from build123d import *

# Parameters (mm, degrees)
SKETCH1_R           = 7
SKETCH1_R_2         = 5
BOSS_EXTRUDE1_DEPTH = 12
CUT_EXTRUDE1_DEPTH  = 40.522145691
FILLET1_R           = 1
BOSS_EXTRUDE2_START = -12
BOSS_EXTRUDE2_DEPTH = 12
FILLET2_R           = 2
CUT_EXTRUDE2_DEPTH  = 59.481408086
SKETCH7_R           = 1.5
CUT_EXTRUDE3_DEPTH  = 65.024019647


with BuildPart() as part:
    # Sketch1 → Boss-Extrude1 (new body)
    with BuildSketch(Plane(origin=(0, 0, 0), x_dir=(0, 0, -1), z_dir=(1, 0, 0))):
        with Locations((-30, 0)):
            Circle(SKETCH1_R)
        with Locations((-30, 0)):
            Circle(SKETCH1_R_2, mode=Mode.SUBTRACT)
    extrude(amount=BOSS_EXTRUDE1_DEPTH)

    # Sketch3 → Cut-Extrude1 (cut, through all)
    with BuildSketch(Plane(origin=(12, 0, 0), x_dir=(0, 0, -1), z_dir=(1, 0, 0))):
        Polygon((-26.132418273, 3.168881756), (-27.092472621, -4.067712446), (-40.54775296, -2.282646151), (-39.587698612, 4.953948051), align=None)
    extrude(amount=-CUT_EXTRUDE1_DEPTH, mode=Mode.SUBTRACT)

    # Fillet1
    fillet1_edges = [part.edges().sort_by_distance(p)[0] for p in [
        (6, 4.067712446, 32.907527379),
        (6, 4.403840469, 35.441156966),
        (6, -3.168881756, 33.867581727),
        (6, -2.832753733, 36.401211314),
    ]]
    fillet(fillet1_edges, radius=FILLET1_R - 0.0001)  # a hair under: the kernel refuses the full size

    # Sketch4 → Boss-Extrude2 (add)
    with BuildSketch(Plane(origin=(12, 0, 0), x_dir=(0, 0, -1), z_dir=(1, 0, 0)).offset(BOSS_EXTRUDE2_START)):
        with BuildLine():
            Line((-23.06080008, -0.92060006), (-17, 40))
            Line((-17, 40), (0, 40))
            Line((0, 40), (0, 45))
            Line((0, 45), (-23, 45))
            Line((-23, 45), (-32.940967226, 6.352221011))
            ThreePointArc((-32.940967226, 6.352221011), (-25.850307511, 5.63737991), (-23.06080008, -0.92060006))
        make_face()
    extrude(amount=BOSS_EXTRUDE2_DEPTH)

    # Fillet2
    fillet2_edges = [part.edges().sort_by_distance(p)[0] for p in [
        (6, 40, 17),
    ]]
    fillet(fillet2_edges, radius=FILLET2_R)

    # Sketch6 → Cut-Extrude2 (cut, through all)
    with BuildSketch(Plane(origin=(12, 0, 0), x_dir=(0, 0, -1), z_dir=(1, 0, 0))):
        with BuildLine():
            Line((-24.037943225, 10.910448491), (-21.102528553, 30.729437441))
            ThreePointArc((-21.102528553, 30.729437441), (-22.170547869, 32.250479964), (-23.74540162, 31.263529469))
            Line((-23.74540162, 31.263529469), (-28.73638424, 11.859945407))
            ThreePointArc((-28.73638424, 11.859945407), (-26.887444194, 8.909635204), (-24.037943225, 10.910448491))
        make_face()
    extrude(amount=-CUT_EXTRUDE2_DEPTH, mode=Mode.SUBTRACT)

    # Mirror9: part across plane


with BuildPart() as part_1:
    add(part.part)
    add(part.part.mirror(Plane(origin=(-56.513793287, 40, 0), x_dir=(1, 0, 0), z_dir=(0, 0, -1))))

    # Sketch7 → Cut-Extrude3 (cut, through all)
    with BuildSketch(Plane(origin=(0, 45, 0), x_dir=(1, 0, 0), z_dir=(0, 1, 0))):
        with Locations(Location((6, -12.5, 0), (0, 0, 270))):
            Circle(SKETCH7_R)
        with Locations(Location((6, 12.5, 0), (0, 0, 270))):
            Circle(SKETCH7_R)
    extrude(amount=-CUT_EXTRUDE3_DEPTH, mode=Mode.SUBTRACT)


solid = part_1.part
Here's how the part is built. I have some questions about the finished solid (model axes, mm). A direction names the side the tool comes from. Coordinates: 2 decimals unless noted, no trailing zeros. Write each loop counter-clockwise with the first axis right and the second up, starting at its lowest first coordinate (ties: lowest second). Pieces come first, ordered by that corner, then holes.
1) If we section it at C-C (y = 0): List the corners of the cut face in (x, z) for me.
Filled in:
outline: (0, -25) - (12, -25) - (12, -22.92) - (0, -22.92) - close; (0, 22.92) - (12, 22.92) - (12, 25) - (0, 25) - close
2) If I drill on line 1 (Z direction, x = 11, y = 25); line 2 (X direction, y = 43.9, z = 12.5); line 3 (Z direction, x = 9, y = 10.5), over which ranges is the centre line in solid material (lowest first)?
Filled in:
line 1: z = -28.14 to -25.36, -21.95 to -19.22, 19.22 to 21.95, 25.36 to 28.14
line 2: x = 0 to 4.5, 7.5 to 12
line 3: z = -31.87 to -28.69, -24.14 to -21.37, 21.37 to 24.14, 28.69 to 31.87
3) Which directions (+Z, -Z, +X, -X, +Y, -Y) give clear straight access to the entire face, cutting with the end or side of a thin tool? Please do faces 5 (the face through (6, 40, 0)), 6 (the face through (6.084, 32.244, -22.142)), 7 (the face through (12, 40.3, -2.8)).
Filled in:
face 5: +X, -X, -Y
face 6: +X, -X
face 7: +Z, -Z, +X, +Y, -Y
4) Thinking about a two-plate mould opening in Y: for faces 1 (the face through (6.084, 21.698, -26.206)), 2 (the face through (6.08, 20.68, 22.59)), 3 (the face through (6, 45, 0)), 4 (the face through (6.1, 39.5, 16.6)), which applies, +Y half, -Y half, draft (parallel to the pull), parting line (faces both ways), or undercut?
Filled in:
face 1: undercut
face 2: undercut
face 3: +Y half
face 4: -Y half
5) If we section it at D-D (y = 26): List the corners of the cut face in (x, z) for me, plus the area to 3 significant figures.
Filled in:
outline: (0, -27.89) - (12, -27.89) - (12, -25.1) - (0, -25.1) - close; (0, -21.8) - (12, -21.8) - (12, -19.07) - (0, -19.07) - close; (0, 19.07) - (12, 19.07) - (12, 21.8) - (0, 21.8) - close; (0, 25.1) - (12, 25.1) - (12, 27.89) - (0, 27.89) - close
area: 132 mm2
6) I'm going to push flat-ended pins straight in: pin 1 (4 mm diameter, centred on x = 2.5, y = 8.5, fed in from +Z); pin 2 (9 mm diameter, centred on y = 0, z = 30, fed in from +X) (1 decimal); pin 3 (3 mm diameter, centred on x = 3.5, y = 38, fed in from -Z); pin 4 (3 mm diameter, centred on x = 5.5, y = 28.5, fed in from -Z). Where does each tip first touch, or does it pass through?
Filled in:
pin 1: stops at z = 32.9
pin 2: passes through
pin 3: stops at z = -25.19
pin 4: stops at z = -27.63
7) If we section it at B-B (x = 10.5): Count the separate pieces of the cut face and the enclosed holes in it, plus the area to 3 significant figures.
Filled in:
separate pieces: 1
enclosed holes: 2
area: 808 mm2
8) If we section it at A-A (z = 12.5): List the corners of the cut face in (x, y) for me, plus the area to 3 significant figures.
Filled in:
outline: (0, 40) - (4.5, 40) - (4.5, 45) - (0, 45) - close; (7.5, 40) - (12, 40) - (12, 45) - (7.5, 45) - close
area: 45.0 mm2
